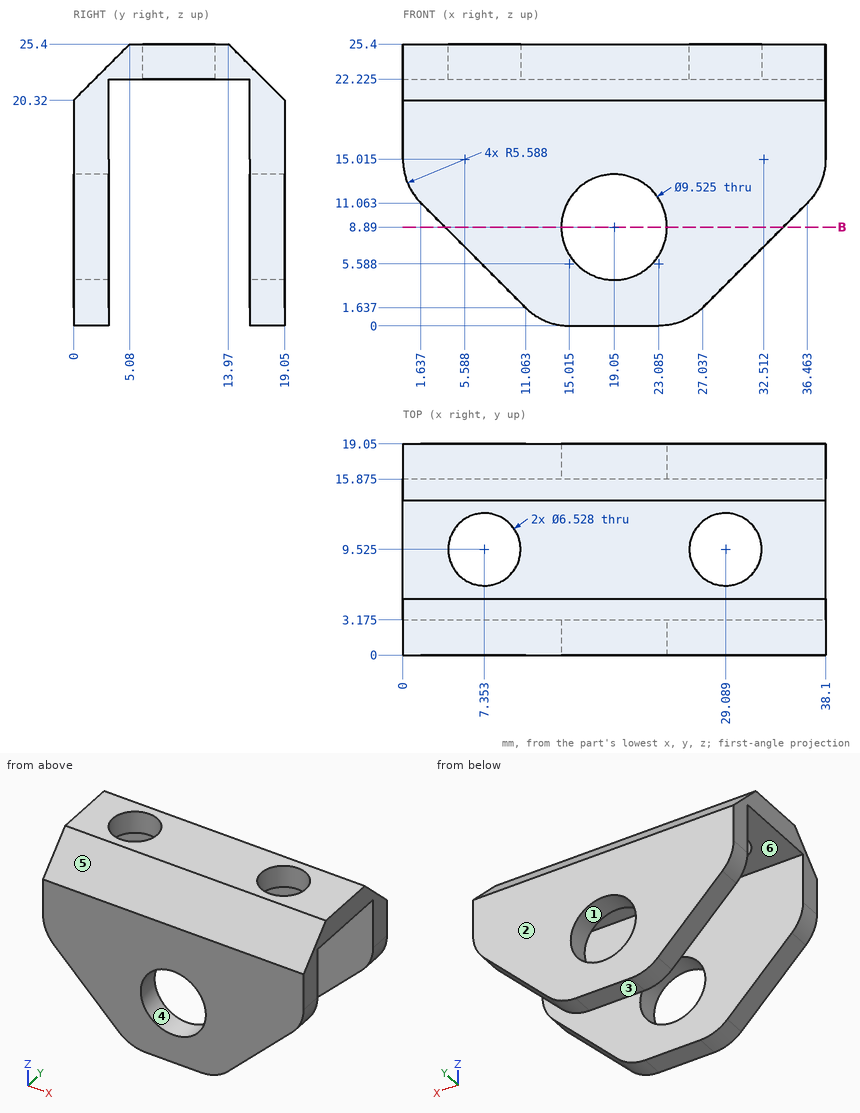
Check sheet for the drawn part. Datum: minimum x, y, z corner. Units: mm. A direction names the side the tool comes from. Coordinates: 2 decimals unless noted, no trailing zeros. Answer as a JSON object with one key per item and string values.
1. Scan lines: L1, parallel to Z at x = 12, y = 13.75 (1 decimal); L2, parallel to Z at x = 19.5, y = 17.75; L3, parallel to Z at x = 23, y = 17.25. Record each from-to range of solid material in increasing order. Write a range as from..to.
Outcome:
{"L1": "22.2..25.4", "L2": "0..4.15, 13.63..21.62", "L3": "0..6.23, 11.55..22.12"}
2. Depth check by flat-ended pin: P1, Ø1.5, axis at x = 7, y = 13, coming from the -Z side (3 decimals); P2, Ø5, axis at x = 20.5, y = 2.5, coming from the +Z side; P3, Ø5, axis at x = 29.09, y = 9.53, coming from the +Z side; P4, Ø1.5, axis at x = 29, y = 4, coming from the +Z side. Enter the tip coordinate at first touch or a pass-through.
Outcome:
{"P1": "z = 22.225", "P2": "z = 25.32", "P3": "through", "P4": "z = 25.07"}
3. Sectioned sample at B-B on z = 8.89. Count the separate pieces of the cut face and the enclosed holes in it, and give its area (3 significant figures).
Outcome:
{"separate pieces": "4", "enclosed holes": "0", "area": "133 mm²"}
4. Release check for a two-part mould opening along Z. For the marked faces 1, 2, 3 and 4 record: pulls with the +Z half, pulls with the -Z half, needs draft (parallel to the pull), parting line crosses it, or undercut.
Outcome:
{"face 1": "undercut", "face 2": "needs draft", "face 3": "pulls with the -Z half", "face 4": "undercut"}
5. Access from +Z, -Z, +X, -X, +Y, -Y to the whole of each face (thin tool, end or side, straight path). Record for the marked faces 5 and 6.
Outcome:
{"face 5": "+Z, +X, -X, -Y", "face 6": "-Z, +X, -X"}
